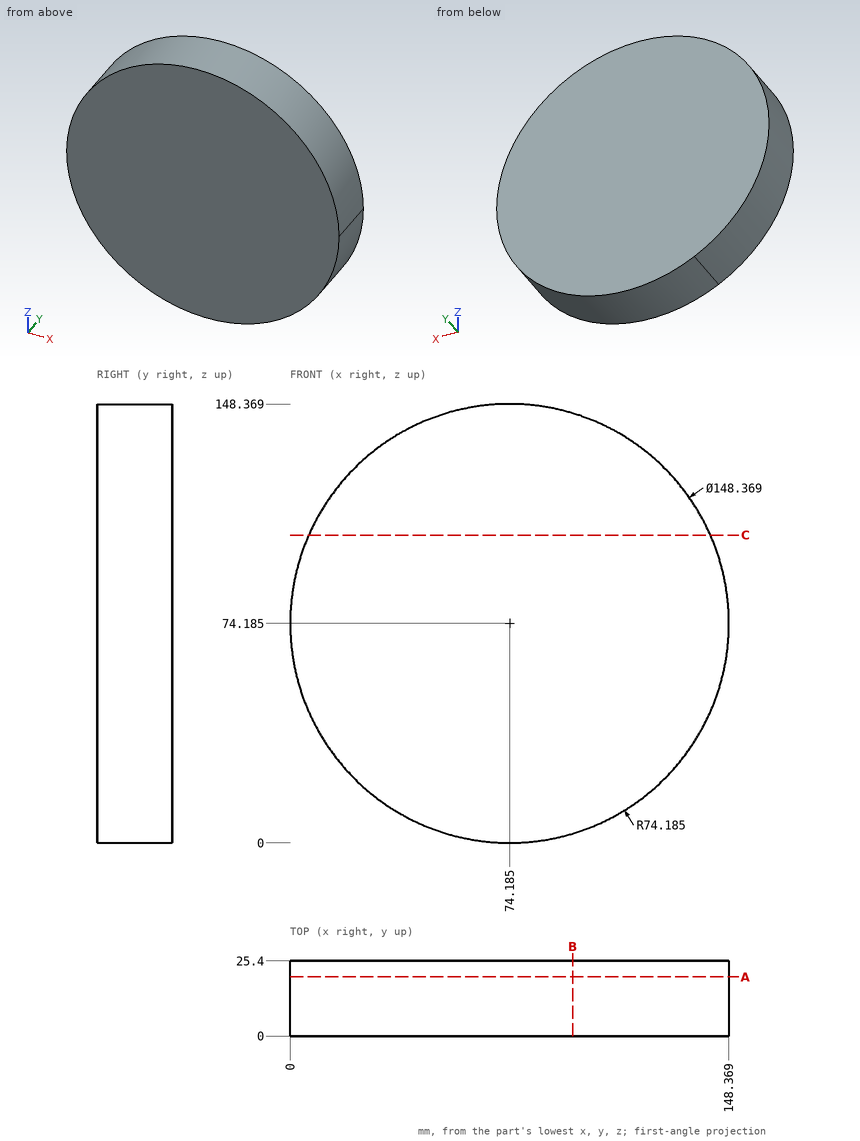
Design review of the part shown in the three views and the two pictorial views. Dimensions are in mm from the part's minimum x, y and z. Give positions to 0.01 mm unless a question says otherwise; leave off trailing zeros. Order: outer loops, then holes, each group sorted by start corner. A loop starts at its lowest first (then second) coordinate and runs counter-clockwise, first axis right, second up. Notation, with made-up numbers: M -37.5,61 L 14.5,61 A21 cw 14.5,66 Z; hole C -22.5,-19.5 d4. An arc over 180 degrees is marked long. Answer in a Markdown table with one row per item. Add a question column.
(1) Wall thickness on probe 1 along Z at (x, y) = (45, 5.5); probe 2 along X at (y, z) = (9.5, 119) (1 decimal); probe 3 along Z at (x, y) = (64, 2.25): over which ranges is each line inside the solid? List them lowest first. Write a range as [from, to].
(2) For pin 1 (10 mm diameter, centred on y = 20.5, z = 119.5, fed in from +X); pin 2 (4 mm diameter, centred on x = 125, y = 9.5, fed in from -Z) (1 decimal); pin 3 (12 mm diameter, centred on x = 126, y = 22, fed in from +Z), all flat-tipped, find the tip position at first contact; note any pin that passes through.
(3) Consider section B-B on x = 95.5. State the section outline as (y, z) points, and give its area (3 significant figures).
(4) Consider section A-A on y = 20. State the section outline as (x, z) points (1 decimal), and give its area (3 significant figures).
(5) Consider section C-C on z = 104. State the section outline as (x, y) points (1 decimal).
Evaluation:
| question | item | result |
|---|---|---|
| 1 | probe 1 | z = [5.98, 142.39] |
| 1 | probe 2 | x = [15.1, 133.3] |
| 1 | probe 3 | z = [0.7, 147.67] |
| 2 | pin 1 | stops at x = 136.46 |
| 2 | pin 2 | stops at z = 18.3 |
| 2 | pin 3 | stops at z = 132.53 |
| 3 | outline | M 0,3.13 L 25.4,3.13 L 25.4,145.24 L 0,145.24 Z |
| 3 | area | 3,610 mm^2 |
| 4 | outline | C 74.2,74.2 d148.4 |
| 4 | area | 17,300 mm^2 |
| 5 | outline | M 6.3,0 L 142.1,0 L 142.1,25.4 L 6.3,25.4 Z |
